Could you check a few things on this model? Use its own coordinates, in mm. Face numbers are marked on the shaded views. A direction names the side the tool comes from. Give positions to 0.01 mm unless a question says otherwise; leave off trailing zeros. Loops run counter-clockwise (first coordinate to the right, second up) from the corner with the lowest first, then second, coordinate; pieces in that order, holes last. Notation, with made-up numbers: (24, 32.5) - (47, 32.5) arc R33 cw to (47, 60.5) - close; hole circle Ø4 at (86, 78). An arc over 180 degrees is marked (long way). Answer in a Markdown table with one row per item. Add a question column.
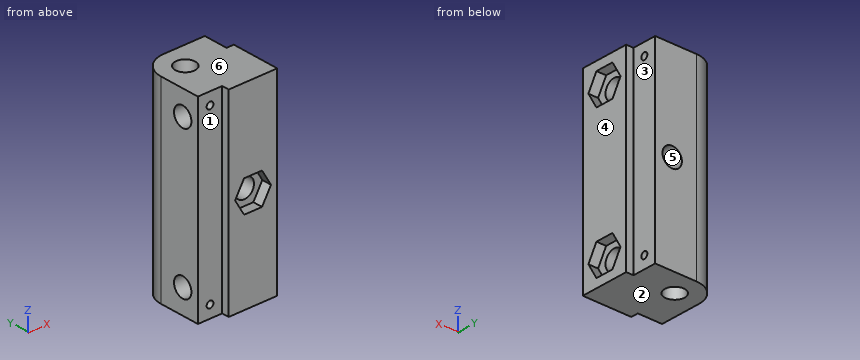
```python
from build123d import *

# Parameters (mm, degrees)
SKETCH004_R  = 1.4
PAD002_DEPTH = 6
SKETCH007_R  = 4
PAD003_DEPTH = 31
SKETCH001_R  = 4
PAD004_DEPTH = 31
SKETCH006_R  = 1.4
PAD005_DEPTH = 5
PAD006_DEPTH = 4
SKETCH003_W  = 10
SKETCH003_H  = 80
PAD007_DEPTH = 3
SKETCH005_W  = 10
SKETCH005_H  = 80
PAD008_DEPTH = 3
PAD001_DEPTH = 4
SKETCH_R     = 4.1
PAD_DEPTH    = 80


with BuildPart() as obj1:
    # Sketch004 → Pad002 (new body)
    with BuildSketch(Plane.YZ.offset(10.029501)):
        with Locations((11.683203, 75)):
            Circle(SKETCH004_R)
        with Locations((11.683203, 5)):
            Circle(SKETCH004_R)
    extrude(amount=-PAD002_DEPTH)


with BuildPart() as rodhole01:
    # Sketch007 → Pad003 (new body)
    with BuildSketch(Plane.XZ.offset(13.316829)):
        with Locations((3.029501, 40)):
            Circle(SKETCH007_R)
    extrude(amount=-PAD003_DEPTH)


with BuildPart() as rodhole02:
    # Sketch001 → Pad004 (new body)
    with BuildSketch(Plane.YZ.offset(13.029501)):
        with Locations((-3.316797, 70)):
            Circle(SKETCH001_R)
        with Locations((-3.316797, 10)):
            Circle(SKETCH001_R)
    extrude(amount=-PAD004_DEPTH)


with BuildPart() as obj2:
    # Sketch006 → Pad005 (new body)
    with BuildSketch(Plane.XZ.offset(10.316829)):
        with Locations((-11.970531, 75)):
            Circle(SKETCH006_R)
        with Locations((-11.970531, 5)):
            Circle(SKETCH006_R)
    extrude(amount=-PAD005_DEPTH)


with BuildPart() as obj3:
    # Sketch002 → Pad006 (new body)
    with BuildSketch(Plane.YZ.offset(13.029501)):
        Polygon((4.083203, 70), (0.383203, 76.408588), (-7.016797, 76.408588), (-10.716797, 70), (-7.016797, 63.591412), (0.383203, 63.591412), align=None)
        Polygon((0.383203, 3.591412), (4.083203, 10), (0.383203, 16.408588), (-7.016797, 16.408588), (-10.716797, 10), (-7.016797, 3.591412), align=None)
    extrude(amount=-PAD006_DEPTH)


with BuildPart() as obj4:
    # Sketch003 → Pad007 (new body)
    with BuildSketch(Plane.YZ.offset(13.029501)):
        with Locations((11.683203, 40)):
            Rectangle(SKETCH003_W, SKETCH003_H)
    extrude(amount=-PAD007_DEPTH)


with BuildPart() as obj5:
    # Sketch005 → Pad008 (new body)
    with BuildSketch(Plane.XZ.offset(13.316829)):
        with Locations((-11.970531, 40)):
            Rectangle(SKETCH005_W, SKETCH005_H)
    extrude(amount=-PAD008_DEPTH)


with BuildPart() as cutblock:
    # Sketch008 → Pad001 (new body)
    with BuildSketch(Plane.XZ.offset(13.316829)):
        Polygon((6.763311, 33.591412), (10.463311, 40), (6.763311, 46.408588), (-0.636689, 46.408588), (-4.336689, 40), (-0.636689, 33.591412), align=None)
    extrude(amount=-PAD001_DEPTH)

    # Fusion: union obj1, RodHole01, RodHole02, obj2, obj3, obj4, obj5
    add(obj1.part)
    add(rodhole01.part)
    add(rodhole02.part)
    add(obj2.part)
    add(obj3.part)
    add(obj4.part)
    add(obj5.part)


with BuildPart() as final:
    # Sketch → Pad (new body)
    with BuildSketch(Plane.XY):
        with BuildLine():
            Line((-16.970531, 6.683171), (-16.970531, -13.316829))
            Line((-16.970531, -13.316829), (13.029501, -13.316829))
            Line((13.029501, -13.316829), (13.029501, 16.683203))
            Line((13.029501, 16.683203), (-6.970499, 16.683203))
            ThreePointArc((-6.970499, 16.683203), (-14.041599, 13.754271), (-16.970531, 6.683171))
        make_face()
        with Locations((-6.970531, 6.683203)):
            Circle(SKETCH_R, mode=Mode.SUBTRACT)
    extrude(amount=PAD_DEPTH)

    # Cut: cut CutBlock
    add(cutblock.part, mode=Mode.SUBTRACT)


solid = final.part
```
(1) For pin 1 Ø8 at (x, z) = (-13.5, 40.5) entering from -Y; pin 2 Ø3 at (x, y) = (4.5, -11.5) entering from -Z; pin 3 Ø2 at (y, z) = (12, 75.5) entering from +X; pin 4 Ø2.5 at (y, z) = (-12, 48) entering from -X, each with a flat end and sliding along its axis, tell me the tip position at first contact or that it passes through.
(2) On a 3-axis mill with a long thin cutter (end or side, diameter ignored), from which of +Z, -Z, +X, -X, +Y, -Y can I reach the whole of each face in a straight line? I mean the marked faces 1, 2 and 3. Say none if no direction works.
(3) I want a section at D-D on y = -1.5. Please give me the cut outline in (x, z).
(4) Please list where these lines run through material, in increasing order: line 1 (Y direction, x = 6, z = 75); line 2 (X direction, y = 9.5, z = 42); line 3 (Z direction, x = -7, y = 0).
(5) I want a section at C-C on z = 72. Please give me the cut outline in (x, y), then the cut area to 3 significant figures.
(6) We'd pull the mould along Z, two halves only. Please class the marked faces 4, 5 and 6: pulls with the +Z half, pulls with the -Z half, needs draft (parallel to the pull), parting line crosses it, or undercut.
(7) I want a section at A-A on z = 28. Please give me the cut outline in (x, y).
(8) I want a section at B-B on x = 5. Please give me the cut outline in (y, z), then the cut area to 3 significant figures.
Reported:
| question | item | result |
|---|---|---|
| 1 | pin 1 | y = -10.32 |
| 1 | pin 2 | z = 0 |
| 1 | pin 3 | x = 10.03 |
| 1 | pin 4 | x = -6.97 |
| 2 | face 1 | +Z, -Z, -X, -Y |
| 2 | face 2 | -Z, +X, -X, +Y, -Y |
| 2 | face 3 | +Z, -Z, +X, +Y |
| 3 | outline | (-16.97, 0) - (13.03, 0) - (13.03, 3.59) - (9.03, 3.59) - (9.03, 6.44) - (-16.97, 6.44) - close; (-16.97, 13.56) - (9.03, 13.56) - (9.03, 16.41) - (13.03, 16.41) - (13.03, 63.59) - (9.03, 63.59) - (9.03, 66.44) - (-16.97, 66.44) - close; (-16.97, 73.56) - (9.03, 73.56) - (9.03, 76.41) - (13.03, 76.41) - (13.03, 80) - (-16.97, 80) - close; hole circle Ø8 at (3.03, 40) |
| 4 | line 1 | -13.32 to 10.28, 13.08 to 16.68 |
| 4 | line 2 | -16.57 to -9.95, -3.99 to -0.43, 6.49 to 10.03 |
| 4 | line 3 | 0 to 7.76, 12.24 to 67.76, 72.24 to 80 |
| 5 | outline | (-16.97, -10.32) - (-6.97, -10.32) - (-6.97, -13.32) - (13.03, -13.32) - (13.03, -9.56) - (9.03, -9.56) - (9.03, -6.78) - (-16.97, -6.78) - close; (-16.97, 0.15) - (9.03, 0.15) - (9.03, 2.93) - (13.03, 2.93) - (13.03, 6.68) - (10.03, 6.68) - (10.03, 16.68) - (-6.97, 16.68) arc R10 ccw to (-16.97, 6.68) - close; hole circle Ø8.2 at (-6.97, 6.68) |
| 5 | area | 536 mm² |
| 6 | face 4 | needs draft |
| 6 | face 5 | undercut |
| 6 | face 6 | pulls with the +Z half |
| 7 | outline | (-16.97, -10.32) - (-6.97, -10.32) - (-6.97, -13.32) - (13.03, -13.32) - (13.03, 6.68) - (10.03, 6.68) - (10.03, 16.68) - (-6.97, 16.68) arc R10 ccw to (-16.97, 6.68) - close; hole circle Ø8.2 at (-6.97, 6.68) |
| 8 | outline | (-13.32, 0) - (16.68, 0) - (16.68, 36.52) - (-9.32, 36.52) - (-9.32, 33.59) - (-13.32, 33.59) - close; (-13.32, 46.41) - (-9.32, 46.41) - (-9.32, 43.48) - (16.68, 43.48) - (16.68, 80) - (-13.32, 80) - close; hole circle Ø8 at (-3.32, 10); hole circle Ø8 at (-3.32, 70); hole circle Ø2.8 at (11.68, 5); hole circle Ø2.8 at (11.68, 75) |
| 8 | area | 2,050 mm² |
